```python
from build123d import *

# Parameters (mm, degrees)
ESQUISSE1_R        = 9
BOSS_EXTRU_1_DEPTH = 1
CHANFREIN1_SIZE    = 0.5
ESQUISSE2_R        = 8
BOSS_EXTRU_2_DEPTH = 3
CHANFREIN2_SIZE    = 0.5


with BuildPart() as part:
    # Esquisse1 → Boss.-Extru.1 (new body)
    with BuildSketch(Plane.XY):
        Circle(ESQUISSE1_R)
    extrude(amount=BOSS_EXTRU_1_DEPTH)

    # Chanfrein1
    chanfrein1_edges = [part.edges().sort_by_distance(p)[0] for p in [
        (-9, 0, 1),
    ]]
    chamfer(chanfrein1_edges, length=CHANFREIN1_SIZE)

    # Esquisse2 → Boss.-Extru.2 (add)
    with BuildSketch(Plane.XY.offset(1)):
        Circle(ESQUISSE2_R)
    extrude(amount=BOSS_EXTRU_2_DEPTH)

    # Chanfrein2
    chanfrein2_edges = [part.edges().sort_by_distance(p)[0] for p in [
        (-8, 0, 4),
    ]]
    chamfer(chanfrein2_edges, length=CHANFREIN2_SIZE)


solid = part.part
```
Input: part model. Units: mm. Frame: model coordinates. A direction names the side the tool comes from. Round coordinates to 2 decimals unless told otherwise and drop trailing zeros. Loops run counter-clockwise (first coordinate to the right, second up) from the corner with the lowest first, then second, coordinate; pieces in that order, holes last.
1) Section query C-C on z = 3.1. Return the cut outline in (x, y).
Ans:
outline: circle Ø16 at (0, 0)
2) Set-up query: faces 1 (the flat face through (0, 0, 0)), 2 (the cylindrical face through (-1.73, -7.81, 2.23)). Return all of +Z, -Z, +X, -X, +Y, -Y with unobstructed straight access to the full face (end or side cutting, diameter ignored); none if empty.
Ans:
face 1: -Z, +X, -X, +Y, -Y
face 2: +Z
3) Material intervals for line 1 (Y direction, x = -0.25, z = 2.55); line 2 (Z direction, x = -4.25, y = 7.25); line 3 (Y direction, x = 6, z = 1.25), sorted ascending.
Ans:
line 1: y = -8 to 8
line 2: z = 0 to 1
line 3: y = -5.29 to 5.29
4) Pin query (flat end, axial travel): pin 1 (1.5 mm diameter, centred on y = -1, z = 3.5, fed in from -X). Return the tip coordinate at first contact, or that it passes through.
Ans:
pin 1: stops at x = -8
5) Section query A-A on y = 0. Return the cut outline in (x, z), plus the area to 3 significant figures.
Ans:
outline: (-9, 0) - (9, 0) - (9, 0.5) - (8.5, 1) - (8, 1) - (8, 3.5) - (7.5, 4) - (-7.5, 4) - (-8, 3.5) - (-8, 1) - (-8.5, 1) - (-9, 0.5) - close
area: 65.5 mm2
